Answer from the drawing. Dimensions are ordinates in mm from the lowest x, y and z of the part. Round coordinates to 2 decimals unless told otherwise and drop trailing zeros. Loops run counter-clockwise (first coordinate to the right, second up) from the corner with the lowest first, then second, coordinate; pieces in that order, holes last.
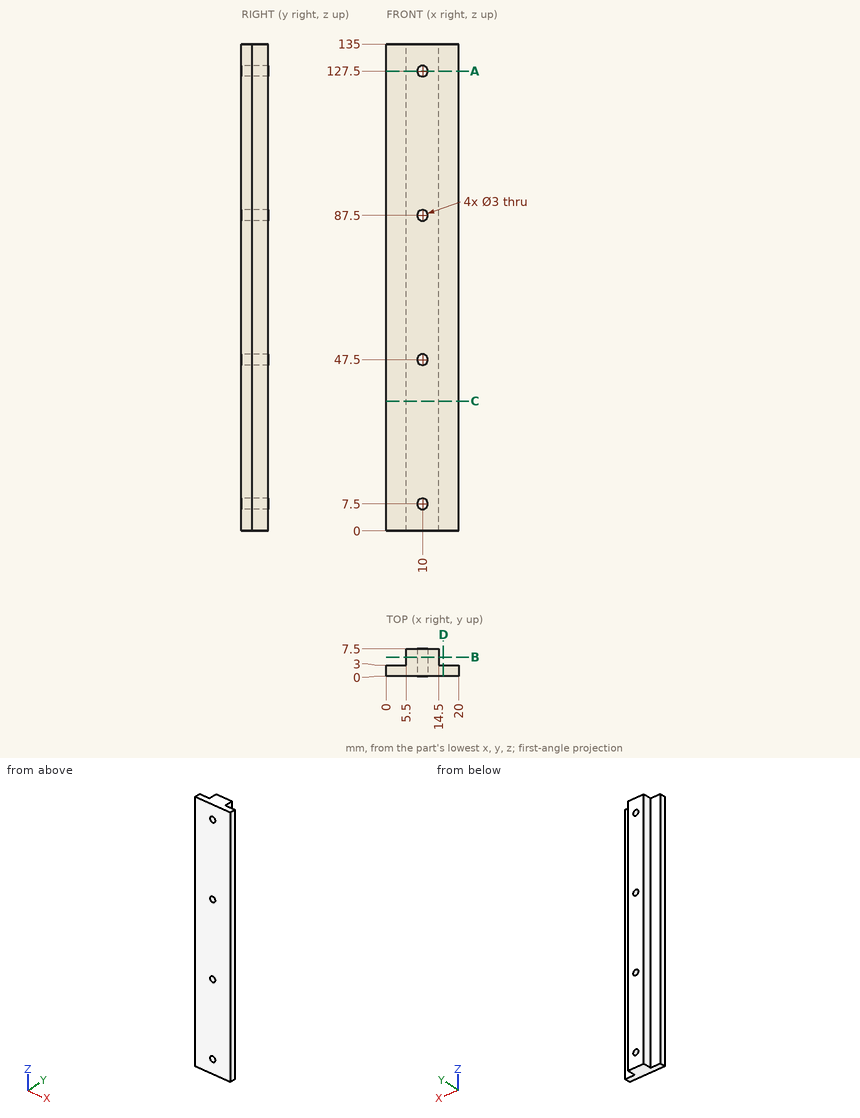
1. Find section B-B (y = 5.25). Write down the section's boundary in (x, z), then the cut area to 3 significant figures.
Answer key:
outline: (5.5, 0) - (14.5, 0) - (14.5, 135) - (5.5, 135) - close; hole circle Ø3 at (10, 7.5); hole circle Ø3 at (10, 47.5); hole circle Ø3 at (10, 87.5); hole circle Ø3 at (10, 127.5)
area: 1,190 mm2
2. Consider probe 1 along Z at (x, y) = (10, 3); probe 2 along X at (y, z) = (6.25, 7.5); probe 3 along Z at (x, y) = (11, 1.25). Determine where each line is inside the solid, lowest interval first.
Answer key:
probe 1: z = 0 to 6, 9 to 46, 49 to 86, 89 to 126, 129 to 135
probe 2: x = 5.5 to 8.5, 11.5 to 14.5
probe 3: z = 0 to 6.38, 8.62 to 46.38, 48.62 to 86.38, 88.62 to 126.38, 128.62 to 135
3. Find section A-A (z = 127.5). Write down the section's boundary in (x, y).
Answer key:
outline: (0, 0) - (8.5, 0) - (8.5, 7.5) - (5.5, 7.5) - (5.5, 3) - (0, 3) - close; (11.5, 0) - (20, 0) - (20, 3) - (14.5, 3) - (14.5, 7.5) - (11.5, 7.5) - close
4. Find section C-C (z = 36). Write down the section's boundary in (x, y), then the cut area to 4 significant figures.
Answer key:
outline: (0, 0) - (20, 0) - (20, 3) - (14.5, 3) - (14.5, 7.5) - (5.5, 7.5) - (5.5, 3) - (0, 3) - close
area: 100.5 mm2
5. Find section D-D (x = 15.75). Write down the section's boundary in (y, z), then the cut area to 3 significant figures.
Answer key:
outline: (0, 0) - (3, 0) - (3, 135) - (0, 135) - close
area: 405 mm2
6. Given pin 1 (1 mm diameter, centred on x = 2.5, z = 33, fed in from +Y); pin 2 (2 mm diameter, centred on y = 4.5, z = 28.5, fed in from -X); pin 3 (2 mm diameter, centred on y = 5.5, z = 83, fed in from +X), each flat-ended and moving along its own axis, determine where each tip first touches the part or whether it passes through.
Answer key:
pin 1: stops at y = 3
pin 2: stops at x = 5.5
pin 3: stops at x = 14.5
